Drawing for the job (mm, zero at the part's lowest x, y, z). A direction names the side the tool comes from. Give positions to 0.01 mm unless a question says otherwise; leave off trailing zeros. Loops run counter-clockwise (first coordinate to the right, second up) from the corner with the lowest first, then second, coordinate; pieces in that order, holes last. Notation, with made-up numbers: M 45.5,51.25 L 90.5,51.25 A15 cw 90.5,60.25 Z; hole C 74.5,77 d2. An arc over 180 degrees is marked long. Use CSV: the item, a comma, the result in double quotes. Start each with the question number.
(1) Two-plate mould, pull along X, no slides. Class the marked faces 3, 4 and 5: pulls with the +X half, pulls with the -X half, needs draft (parallel to the pull), parting line crosses it, or undercut.
(2) Slice it at C-C on z = 56.5. State how many separate pieces and enclosed holes the cut face has, and give its area (3 significant figures).
(3) Tool access for the marked faces 1 and 2: list every direction of +Z, -Z, +X, -X, +Y, -Y with a clear straight run to the whole face (end or side of a thin tool).
(4) Slice it at A-A on y = 173. List the corners of the cut face in (x, z).
(5) Wall check: line 1 along X through (y, z) = (100.5, 168) (3 decimals); line 2 along X through (y, z) = (161.5, 200.5); line 3 along Y through (x, z) = (38.5, 291.5). Give the ranges that are in metal, low to high. Write a range as from..to.
(6) Flat gauge pin, fed straight in: P1, Ø12, axis at x = 219, z = 60.5, coming from the +Y side. Where does the tip first touch, or does it go through?
(7) Slice it at B-B on x = 117.5. List the corners of the cut face in (y, z).
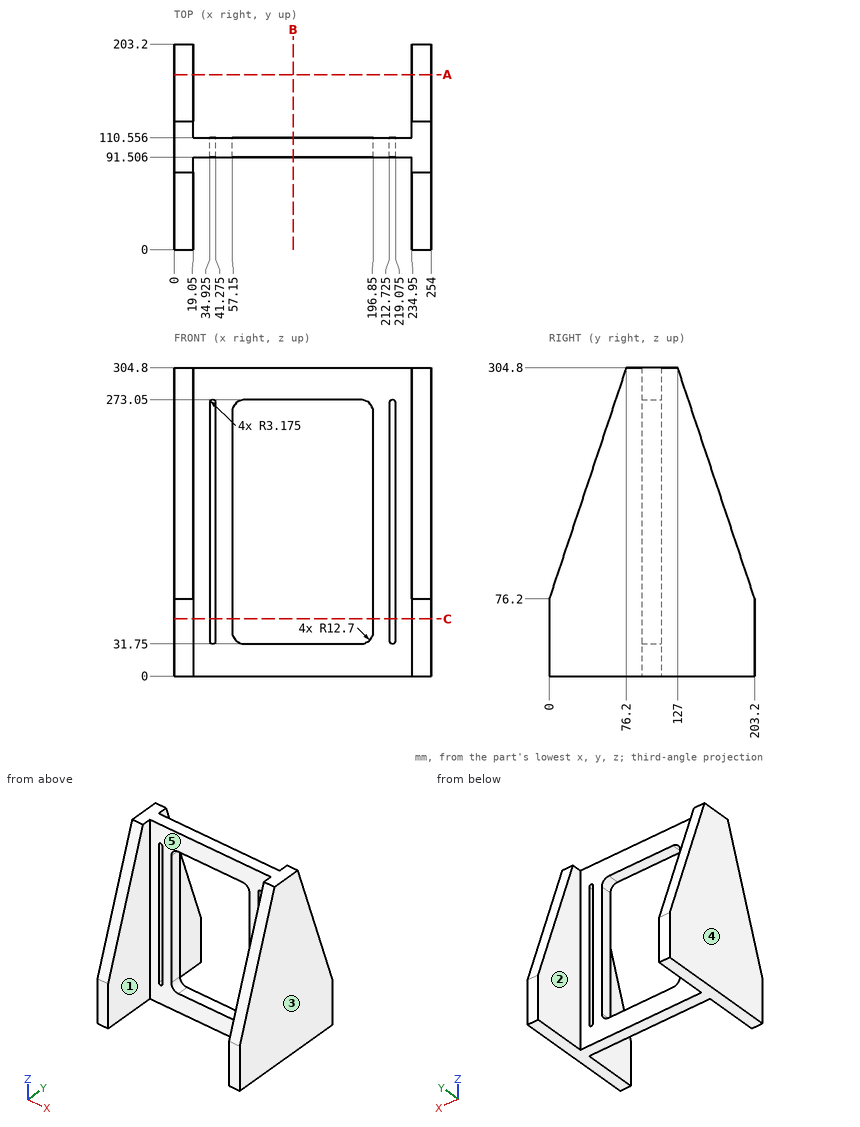
Reply:
1,face 3,"pulls with the +X half"
1,face 4,"pulls with the -X half"
1,face 5,"undercut"
2,separate pieces,"4"
2,enclosed holes,"0"
2,area,"8,950 mm^2"
3,face 1,"+Z, -Z, -Y"
3,face 2,"+Z, -Z, +Y"
4,outline,"M 0,0 L 19.05,0 L 19.05,166.8 L 0,166.8 Z; M 234.95,0 L 254,0 L 254,166.8 L 234.95,166.8 Z"
5,line 1,"x = 0..34.925, 41.275..57.15, 196.85..212.725, 219.075..254"
5,line 2,"x = 0..19.05, 234.95..254"
5,line 3,"y = 91.51..110.56"
6,P1,"stops at y = 110.56"
7,outline,"M 91.51,0 L 110.56,0 L 110.56,31.75 L 91.51,31.75 Z; M 91.51,273.05 L 110.56,273.05 L 110.56,304.8 L 91.51,304.8 Z"
